```python
from build123d import *

# Parameters (mm, degrees)
SKETCH1_W                      = 32
SKETCH1_H                      = 32
BOSS_EXTRUDE1_DEPTH            = 6
SKETCH2_W                      = 10.5
SKETCH2_H                      = 50
F_4_4_4_4_DIAMETER_HOLE1_D     = 4.4
F_4_4_4_4_DIAMETER_HOLE1_DEPTH = 56
HOLE1_D                        = 12.05
FILLET1_R                      = 1


with BuildPart() as part:
    # Sketch1 → Boss-Extrude1 (new body)
    with BuildSketch(Plane.XZ):
        with Locations((16, -16)):
            Rectangle(SKETCH1_W, SKETCH1_H)
    extrude(amount=-BOSS_EXTRUDE1_DEPTH)

    # Sketch2 → Revolve1 (revolve)
    with BuildSketch(Plane(origin=(0, 0, -16.000000238), x_dir=(-1, 0, 0), z_dir=(0, 0, -1)), mode=Mode.PRIVATE) as revolve1_sk:
        with Locations((-21.250000238, 31)):
            Rectangle(SKETCH2_W, SKETCH2_H)
    revolve(revolve1_sk.sketch.rotate(Axis((16.000000238, 6, -16.000000238), (0, 1, 0)), 270), axis=Axis((16.000000238, 6, -16.000000238), (0, 1, 0)))

    # Ø4.4 (4.4) Diameter Hole1
    with Locations(Plane(origin=(0, 0, 0), x_dir=(-1, 0, 0), z_dir=(0, -1, 0))):
        with Locations((-28, 4), (-28, 28), (-4.00000006, 4.00000006), (-4.00000006, 28.000000417)):
            Hole(F_4_4_4_4_DIAMETER_HOLE1_D / 2, depth=F_4_4_4_4_DIAMETER_HOLE1_DEPTH)

    # Hole1 (through all)
    with Locations(Plane(origin=(0, 56, 0), x_dir=(1, 0, 0), z_dir=(0, 1, 0))):
        with Locations((16.000000238, 16.000000238)):
            Hole(HOLE1_D / 2)

    # Fillet1
    fillet1_edges = [part.edges().sort_by_distance(p)[0] for p in [
        (0, 3, -32),
        (0, 3, 0),
        (32, 3, 0),
        (32, 3, -32),
    ]]
    fillet(fillet1_edges, radius=FILLET1_R)


solid = part.part
```
Verification items for the finished model (mm, model axes). A direction names the side the tool comes from. Round coordinates to 2 decimals unless told otherwise and drop trailing zeros. Write each loop counter-clockwise with the first axis right and the second up, starting at its lowest first coordinate (ties: lowest second). Pieces come first, ordered by that corner, then holes.
1. Section check B-B on x = 16. Enter the section's corners in (y, z) (3 decimals).
2. Access from +Z, -Z, +X, -X, +Y, -Y to the whole of each face (thin tool, end or side, straight path). Record for faces 4 (the flat face through (0, 3, -16)), 5 (the flat face through (16, 6, -5)).
3. Section check D-D on x = 4. Enter the section's corners in (y, z), plus the area to 3 significant figures.
4. Section check C-C on z = -16. Enter the section's corners in (x, y) (3 decimals), plus the area to 3 significant figures.
5. Draft check along X on faces 1 (the cylindrical face through (27.523, 3.042, -25.852)), 2 (the flat face through (16, 3, 0)), 3 (the cylindrical face through (26.41, 31.35, -17.37)). Enter one of: +X half, -X half, draft (parallel to the pull), parting line (faces both ways), or undercut.
6. Section check A-A on z = -28. Enter the section's corners in (x, y), plus the area to 3 significant figures.
7. Gauge pin test, flat ends, axial feed: P1, Ø6, axis at y = 38, z = -17.5, coming from the -X side; P2, Ø1.5, axis at x = 9, y = 45, coming from the -Z side; P3, Ø6, axis at y = 49.5, z = -22.5, coming from the +X side. Record the tip position at first contact, or that the pin passes through.
8. Scan lines: L1, parallel to Z at x = 4, y = 4; L2, parallel to X at y = 21, z = -16 (3 decimals); L3, parallel to Z at x = 17, y = 41. Record each from-to range of solid material in increasing order.
Answer:
1. outline: (0, -32) - (6, -32) - (6, -26.5) - (56, -26.5) - (56, -22.025) - (0, -22.025) - close; (0, -9.975) - (56, -9.975) - (56, -5.5) - (6, -5.5) - (6, 0) - (0, 0) - close
2. face 4: +Z, -Z, -X, +Y, -Y
2. face 5: +Y
3. outline: (0, -32) - (6, -32) - (6, -30.2) - (0, -30.2) - close; (0, -25.8) - (6, -25.8) - (6, -6.2) - (0, -6.2) - close; (0, -1.8) - (6, -1.8) - (6, 0) - (0, 0) - close
3. area: 139 mm2
4. outline: (0, 0) - (9.975, 0) - (9.975, 56) - (5.5, 56) - (5.5, 6) - (0, 6) - close; (22.025, 0) - (32, 0) - (32, 6) - (26.5, 6) - (26.5, 56) - (22.025, 56) - close
4. area: 567 mm2
5. face 1: undercut
5. face 2: draft
5. face 3: parting line
6. outline: (0, 0) - (1.8, 0) - (1.8, 6) - (0, 6) - close; (6.2, 0) - (25.8, 0) - (25.8, 6) - (6.2, 6) - close; (30.2, 0) - (32, 0) - (32, 6) - (30.2, 6) - close
6. area: 139 mm2
7. P1: stops at x = 5.5
7. P2: stops at z = -24.44
7. P3: stops at x = 25.9
8. L1: z = -32 to -30.2, -25.8 to -6.2, -1.8 to 0
8. L2: x = 5.5 to 9.975, 22.025 to 26.5
8. L3: z = -26.45 to -21.94, -10.06 to -5.55
